Autodesk Fusion 360 part; units mm, degrees
sketch "Sketch2" plane through (0, 0, 0) normal (0, 0, 1) x (1, 0, 0)
  line L0 (91, -8) -> (-31, -8)
  line L1 (-10, 2.005) -> (70, 2.005)
  line L2 (70, 2.005) -> (77.9321, 7.0743)
  line L3 (-10, 2.005) -> (-17.9321, 7.0743)
  arc A0 (-17.9321, 7.0743) -> (-31, -8) centre (-25, 0) ccw
  arc A1 (91, -8) -> (77.9321, 7.0743) centre (85, 0) ccw
  dimension "d20" = 20
  dimension "d21" = 20
  dimension "d22" = 110
  dimension "d24" = 10.005
extrude "Extrude1" add sketch "Sketch2" along normal blind 8
sketch "Sketch3" plane through (0, 0, 8) normal (0, 0, 1) x (-1, 0, 0)
  line L0 (10, -2.005) -> (17.9321, -7.0743)
  arc A0 (17.9321, -7.0743) -> (31, 8) centre (25, 0) ccw
  line L1 (31, 8) -> (-91, 8)
  arc A1 (-91, 8) -> (-77.9321, -7.0743) centre (-85, 0) ccw
  line L2 (-77.9321, -7.0743) -> (-70, -2.005)
  line L3 (-70, -2.005) -> (10, -2.005)
  circle A2 centre (-85, 0) radius 6.1
  dimension "d28" = 12.2
sketch "Sketch4" plane through (0, 0, 0) normal (0, 0, -1) x (1, 0, 0)
  line L0 (-17.9321, -7.0743) -> (-10, -2.005)
  line L1 (-10, -2.005) -> (70, -2.005)
  line L2 (70, -2.005) -> (77.9321, -7.0743)
  arc A0 (77.9321, -7.0743) -> (91, 8) centre (85, 0) ccw
  line L3 (91, 8) -> (-31, 8)
  arc A1 (-31, 8) -> (-17.9321, -7.0743) centre (-25, 0) ccw
  circle A2 centre (-25, 0) radius 6.1
  dimension "d32" = 12.2
extrude "Extrude4" cut sketch "Sketch4" against normal blind 1.5 contours A2
extrude "Extrude5" cut sketch "Sketch3" against normal blind 1.5 contours A2
sketch "Sketch5" plane through (0, 0, 0) normal (0, 0, -1) x (1, 0, 0)
  circle A0 centre (-25, 0) radius 6.1
  line L0 (-17.9321, -7.0743) -> (-10, -2.005)
  line L1 (-10, -2.005) -> (70, -2.005)
  line L2 (70, -2.005) -> (77.9321, -7.0743)
  arc A1 (77.9321, -7.0743) -> (91, 8) centre (85, 0) ccw
  line L3 (91, 8) -> (-31, 8)
  arc A2 (-31, 8) -> (-17.9321, -7.0743) centre (-25, 0) ccw
  circle A3 centre (85, 0) radius 1.5
  dimension "d39" = 3
extrude "Extrude7" cut sketch "Sketch5" against normal blind 13 contours A3
sketch "Sketch6" plane through (0, 0, 8) normal (0, 0, 1) x (-1, 0, 0)
  circle A0 centre (-85, 0) radius 6.1
  line L0 (10, -2.005) -> (17.9321, -7.0743)
  arc A1 (17.9321, -7.0743) -> (31, 8) centre (25, 0) ccw
  line L1 (31, 8) -> (-91, 8)
  arc A2 (-91, 8) -> (-77.9321, -7.0743) centre (-85, 0) ccw
  line L2 (-77.9321, -7.0743) -> (-70, -2.005)
  line L3 (-70, -2.005) -> (10, -2.005)
  circle A3 centre (25, 0) radius 1.5
  dimension "d44" = 3
extrude "Extrude8" cut sketch "Sketch6" against normal blind 11 contours A3
component "arm1" placed x (1, 0, 0) y (0, 1, 0) z (0, 0, 1) at (0, 0, 0)
Can you work these out from the model? Positions are in its coordinate system, mm. A direction names the side the tool comes from. Coordinates: 2 decimals unless noted, no trailing zeros. Loops run counter-clockwise (first coordinate to the right, second up) from the corner with the lowest first, then second, coordinate; pieces in that order, holes last.
1) For pin 1 (3 mm diameter, centred on y = 2.5, z = 4.5, fed in from +X); pin 2 (1 mm diameter, centred on y = -1.5, z = 3, fed in from -X); pin 3 (4 mm diameter, centred on x = 51, z = 4, fed in from +Y) (3 decimals); pin 4 (1.8 mm diameter, centred on x = -25, y = 0, fed in from -Z), each with a flat end and sliding along its axis, tell me the tip position at first contact or that it passes through.
2) Imagine slicing it at B-B on z = 3.5. List the corners of the cut face in (x, y) for me (3 decimals), plus the area to 3 significant figures.
3) Thinking about a two-plate mould opening in X: for faces 1 (the flat face through (29, 2.005, 4)), 2 (the flat face through (31, -8, 4)), which applies, pulls with the +X half, pulls with the -X half, needs draft (parallel to the pull), parting line crosses it, or undercut?
4) Imagine slicing it at A-A on x = 85. List the corners of the cut face in (y, z) for me, plus the area to 3 significant figures.
5) Imagine slicing it at D-D on x = 18. List the corners of the cut face in (y, z) for me (3 decimals), plus the area to 3 significant figures.
6) I need wall thicknesses on probe 1 along X at (y, z) = (0, 7.1); probe 2 along X at (y, z) = (0, 5.75); probe 3 along Y at (x, z) = (-25, 0.4). Which ranges of each line are inside material? Lowest first, please.
7) Imagine slicing it at C-C on y = 0. List the corners of the cut face in (x, z) for me.
8) Which directions (+Z, -Z, +X, -X, +Y, -Y) give clear straight access to the entire face, cutting with the end or side of a thin tool? Please do faces 3 (the cylindrical face through (-33, 6, 4)), 4 (the flat face through (-13.911, 4.504, 3.944)), 5 (the cylindrical face through (79.365, 2.336, 7.26)), 6 (the cylindrical face through (-31.094, -0.268, 0.74)), 7 (the flat face through (29, -1, 8)).
Completed:
1. pin 1: stops at x = 94.95
1. pin 2: stops at x = -34.95
1. pin 3: stops at y = 2.005
1. pin 4: passes through
2. outline: (-31, -8) - (91, -8) arc R10 ccw (long way) to (77.932, 7.074) - (70, 2.005) - (-10, 2.005) - (-17.932, 7.074) arc R10 ccw (long way) to start; hole circle Ø3 at (-25, 0); hole circle Ø3 at (85, 0)
2. area: 1,520 mm2
3. face 1: undercut
3. face 2: needs draft
4. outline: (-8, 0) - (-1.5, 0) - (-1.5, 6.5) - (-6.1, 6.5) - (-6.1, 8) - (-8, 8) - close; (1.5, 0) - (10, 0) - (10, 8) - (6.1, 8) - (6.1, 6.5) - (1.5, 6.5) - close
4. area: 106 mm2
5. outline: (-8, 0) - (2.005, 0) - (2.005, 8) - (-8, 8) - close
5. area: 80.0 mm2
6. probe 1: x = -35 to -26.5, -23.5 to 78.9, 91.1 to 95
6. probe 2: x = -35 to -26.5, -23.5 to 83.5, 86.5 to 95
6. probe 3: y = -8 to -6.1, 6.1 to 10
7. outline: (-35, 0) - (-31.1, 0) - (-31.1, 1.5) - (-26.5, 1.5) - (-26.5, 8) - (-35, 8) - close; (-23.5, 1.5) - (-18.9, 1.5) - (-18.9, 0) - (83.5, 0) - (83.5, 6.5) - (78.9, 6.5) - (78.9, 8) - (-23.5, 8) - close; (86.5, 0) - (95, 0) - (95, 8) - (91.1, 8) - (91.1, 6.5) - (86.5, 6.5) - close
8. face 3: +Z, -Z
8. face 4: +Z, -Z, +Y
8. face 5: +Z
8. face 6: -Z
8. face 7: +Z, +X, -X, +Y, -Y
